Source: CAD feature listing. Evaluate the final solid. Frame: model axes, mm. Face numbers are marked on the shaded views. A direction names the side the tool comes from. Coordinates: 2 decimals unless noted, no trailing zeros. Loops run counter-clockwise (first coordinate to the right, second up) from the corner with the lowest first, then second, coordinate; pieces in that order, holes last.
from build123d import *

# Parameters (mm, degrees)
F3_DEPTH = 50.801


with BuildPart() as f1:
    # F0 (on Front) → F1 (revolve)
    with BuildSketch(Plane.XZ):
        Polygon((0, 76.2), (0, 25.4), (69.85, 25.4), (69.85, 63.5), (50.8, 63.5), (50.8, 139.7), (12.7, 139.7), (12.7, 76.2), align=None)
    revolve(axis=Axis((-2.3766048754, 0, 0), (1, 0, 0)))

    # F2 (on face) → F3 (cut, through all)
    with BuildSketch(Plane.YZ.offset(50.8)):
        with BuildLine():
            ThreePointArc((9.5145297678, 101.153515625), (0, 101.6), (-9.5145297678, 101.153515625))
            ThreePointArc((-9.5145297678, 101.153515625), (0, 92.075), (9.5145297678, 101.153515625))
        make_face()
        with BuildLine():
            ThreePointArc((9.5145297678, 101.153515625), (9.5223820822, 101.3766964382), (9.525, 101.6))
            ThreePointArc((9.525, 101.6), (-0.2233035618, 111.1223820822), (-9.5145297678, 101.153515625))
            ThreePointArc((-9.5145297678, 101.153515625), (0, 101.6), (9.5145297678, 101.153515625))
        make_face()
        with BuildLine():
            ThreePointArc((-62.3170489686, 71.8420489686), (-62.9590604886, 75.2798012378), (-64.7985483207, 78.2541253579))
            ThreePointArc((-64.7985483207, 78.2541253579), (-71.8420489686, 71.8420489686), (-78.2541253579, 64.7985483207))
            ThreePointArc((-78.2541253579, 64.7985483207), (-67.9916855187, 63.1299696356), (-62.3170489686, 71.8420489686))
        make_face()
        with BuildLine():
            ThreePointArc((-78.2541253579, 64.7985483207), (-71.8420489686, 71.8420489686), (-64.7985483207, 78.2541253579))
            ThreePointArc((-64.7985483207, 78.2541253579), (-78.5772410594, 78.5772410594), (-78.2541253579, 64.7985483207))
        make_face()
        with BuildLine():
            ThreePointArc((-92.075, 0), (-94.7087595938, 6.5754414805), (-101.153515625, 9.5145297678))
            ThreePointArc((-101.153515625, 9.5145297678), (-101.6, 0), (-101.153515625, -9.5145297678))
            ThreePointArc((-101.153515625, -9.5145297678), (-94.7087595938, -6.5754414805), (-92.075, 0))
        make_face()
        with BuildLine():
            ThreePointArc((-101.153515625, -9.5145297678), (-101.6, 0), (-101.153515625, 9.5145297678))
            ThreePointArc((-101.153515625, 9.5145297678), (-111.125, 0), (-101.153515625, -9.5145297678))
        make_face()
        with BuildLine():
            ThreePointArc((-64.7985483207, -78.2541253579), (-71.8420489686, -71.8420489686), (-78.2541253579, -64.7985483207))
            ThreePointArc((-78.2541253579, -64.7985483207), (-78.5772410594, -78.5772410594), (-64.7985483207, -78.2541253579))
        make_face()
        with BuildLine():
            ThreePointArc((-62.3170489686, -71.8420489686), (-67.9916855187, -63.1299696356), (-78.2541253579, -64.7985483207))
            ThreePointArc((-78.2541253579, -64.7985483207), (-71.8420489686, -71.8420489686), (-64.7985483207, -78.2541253579))
            ThreePointArc((-64.7985483207, -78.2541253579), (-62.9590604886, -75.2798012378), (-62.3170489686, -71.8420489686))
        make_face()
        with BuildLine():
            ThreePointArc((9.5145297678, -101.153515625), (0, -92.075), (-9.5145297678, -101.153515625))
            ThreePointArc((-9.5145297678, -101.153515625), (0, -101.6), (9.5145297678, -101.153515625))
        make_face()
        with BuildLine():
            ThreePointArc((9.5145297678, -101.153515625), (0, -101.6), (-9.5145297678, -101.153515625))
            ThreePointArc((-9.5145297678, -101.153515625), (-0.2233035618, -111.1223820822), (9.525, -101.6))
            ThreePointArc((9.525, -101.6), (9.5223820822, -101.3766964382), (9.5145297678, -101.153515625))
        make_face()
        with BuildLine():
            ThreePointArc((81.3670489686, -71.8420489686), (80.5541283015, -67.9916855187), (78.2541253579, -64.7985483207))
            ThreePointArc((78.2541253579, -64.7985483207), (71.8420489686, -71.8420489686), (64.7985483207, -78.2541253579))
            ThreePointArc((64.7985483207, -78.2541253579), (75.2798012378, -80.7250374485), (81.3670489686, -71.8420489686))
        make_face()
        with BuildLine():
            ThreePointArc((64.7985483207, -78.2541253579), (71.8420489686, -71.8420489686), (78.2541253579, -64.7985483207))
            ThreePointArc((78.2541253579, -64.7985483207), (65.1068568778, -65.1068568778), (64.7985483207, -78.2541253579))
        make_face()
        with BuildLine():
            ThreePointArc((101.6, 0), (101.4883175235, 4.7625), (101.153515625, 9.5145297678))
            ThreePointArc((101.153515625, 9.5145297678), (92.075, 0), (101.153515625, -9.5145297678))
            ThreePointArc((101.153515625, -9.5145297678), (101.4883175235, -4.7625), (101.6, 0))
        make_face()
        with BuildLine():
            ThreePointArc((111.125, 0), (108.1754414805, 6.8912404062), (101.153515625, 9.5145297678))
            ThreePointArc((101.153515625, 9.5145297678), (101.4883175235, 4.7625), (101.6, 0))
            ThreePointArc((101.6, 0), (101.4883175235, -4.7625), (101.153515625, -9.5145297678))
            ThreePointArc((101.153515625, -9.5145297678), (108.1754414805, -6.8912404062), (111.125, 0))
        make_face()
        with BuildLine():
            ThreePointArc((81.3670489686, 71.8420489686), (75.2798012378, 80.7250374485), (64.7985483207, 78.2541253579))
            ThreePointArc((64.7985483207, 78.2541253579), (71.8420489686, 71.8420489686), (78.2541253579, 64.7985483207))
            ThreePointArc((78.2541253579, 64.7985483207), (80.5541283015, 67.9916855187), (81.3670489686, 71.8420489686))
        make_face()
        with BuildLine():
            ThreePointArc((78.2541253579, 64.7985483207), (71.8420489686, 71.8420489686), (64.7985483207, 78.2541253579))
            ThreePointArc((64.7985483207, 78.2541253579), (65.1068568778, 65.1068568778), (78.2541253579, 64.7985483207))
        make_face()
    extrude(amount=-F3_DEPTH, mode=Mode.SUBTRACT)


solid = f1.part
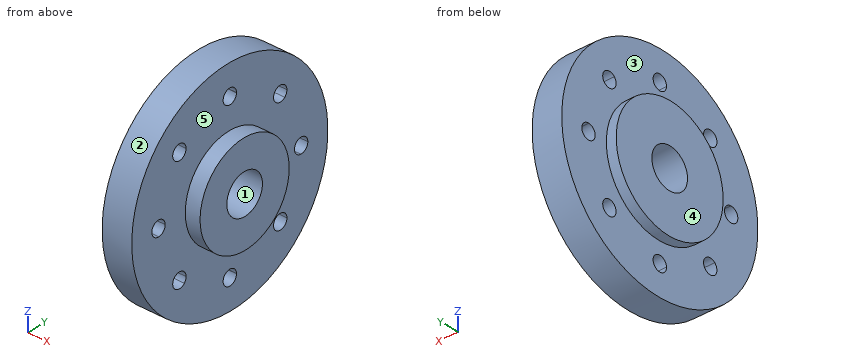
Q1. Section B-B, the plane x = 43.5. Count the separate pieces of the cut face and the enclosed holes in it, plus the area to 3 significant figures.
Q2. Section D-D, the plane x = 64. Return the cut outline in (y, z), plus the area to 3 significant figures.
Q3. Section A-A, the plane y = 0. Return the cut outline in (x, z) (3 decimals), plus the area to 4 significant figures.
Q4. Contact query for flat-ended pins moving along their axis: pin 1 Ø2 at (x, y) = (21.5, 78.5) entering from -Z; pin 2 Ø2 at (x, z) = (59.5, 53) entering from +Y; pin 3 Ø2 at (x, z) = (58, -37) entering from +Y. Output: stop coordinate, or through.
Q5. Section C-C, the plane z = 31.5. Return the cut outline in (x, y).
Q6. Line query: line 1 along Y through (x, z) = (52.5, 0); line 2 along X through (y, z) = (87, -70.5). Output: solid intervals per line, ascending.
Q7. Access query for the marked faces 4 and 5. Directions: +Z, -Z, +X, -X, +Y, -Y. A direction counts if a zero-diameter tool reaches every point of the face in a straight line with its end or side. Return the directions, or none.
Q8. Draft query along Z for the marked faces 1, 2 and 3. Return one class per face: +Z half, -Z half, draft (parallel to the pull), parting line (faces both ways), or undercut.
Derived:
1. separate pieces: 1
1. enclosed holes: 9
1. area: 57,000 mm2
2. outline: circle Ø127 at (0, 0); hole circle Ø50.8 at (0, 0)
2. area: 10,600 mm2
3. outline: (0, -76.2) - (12.7, -76.2) - (12.7, -92.075) - (50.8, -92.075) - (50.8, -63.5) - (69.85, -63.5) - (69.85, -25.4) - (0, -25.4) - close; (0, 25.4) - (69.85, 25.4) - (69.85, 63.5) - (50.8, 63.5) - (50.8, 92.075) - (12.7, 92.075) - (12.7, 76.2) - (0, 76.2) - close; (12.7, -139.7) - (50.8, -139.7) - (50.8, -111.125) - (12.7, -111.125) - close; (12.7, 111.125) - (50.8, 111.125) - (50.8, 139.7) - (12.7, 139.7) - close
3. area: 10,000 mm2
4. pin 1: stops at z = -116.23
4. pin 2: stops at y = 36.45
4. pin 3: stops at y = 52.31
5. outline: (0, -69.38) - (12.7, -69.38) - (12.7, -136.1) - (50.8, -136.1) - (50.8, -55.14) - (69.85, -55.14) - (69.85, 55.14) - (50.8, 55.14) - (50.8, 136.1) - (12.7, 136.1) - (12.7, 69.38) - (0, 69.38) - close
6. line 1: y = -63.5 to -25.4, 25.4 to 63.5
6. line 2: x = 12.7 to 50.8
7. face 4: +Z, -Z, -X, +Y, -Y
7. face 5: +X
8. face 1: undercut
8. face 2: parting line
8. face 3: draft
